Study the drawing (mm; zero at the part's minimum x, y, z) and answer. Round coordinates to 2 decimals unless told otherwise and drop trailing zeros. Loops run counter-clockwise (first coordinate to the right, second up) from the corner with the lowest first, then second, coordinate; pieces in that order, holes last. Notation, with made-up numbers: (58.25, -2) -> (71.25, -2) arc R26 cw to (71.25, 21) -> close; hole circle Ø4 at (-4, 17). An arc over 180 degrees is marked (long way). Write each question's results on one line, items separated by ' | '. Start each with the question number.
(1) The part is cut by section A-A (y = 2.5). Count the separate pieces of the cut face and the enclosed holes in it, plus the area to 3 significant figures.
(2) The part is cut by section D-D (z = 36). Determine the outline of the cut face in (x, y).
(3) The part is cut by section C-C (z = 12.7). Determine the outline of the cut face in (x, y).
(4) Straight lines are drawn through the part: probe 1 along X at (y, z) = (2, 38.1); probe 2 along Z at (x, y) = (19.5, 4.25) (1 decimal); probe 3 along Z at (x, y) = (21.5, 5.5) (1 decimal). For each, find the intervals that lie inside material, in ascending order.
(5) Determine the mould class of the marked faces 1 and 2 for opening direction X: released by +X, released by -X, zero draft, split by the parting line, or undercut.
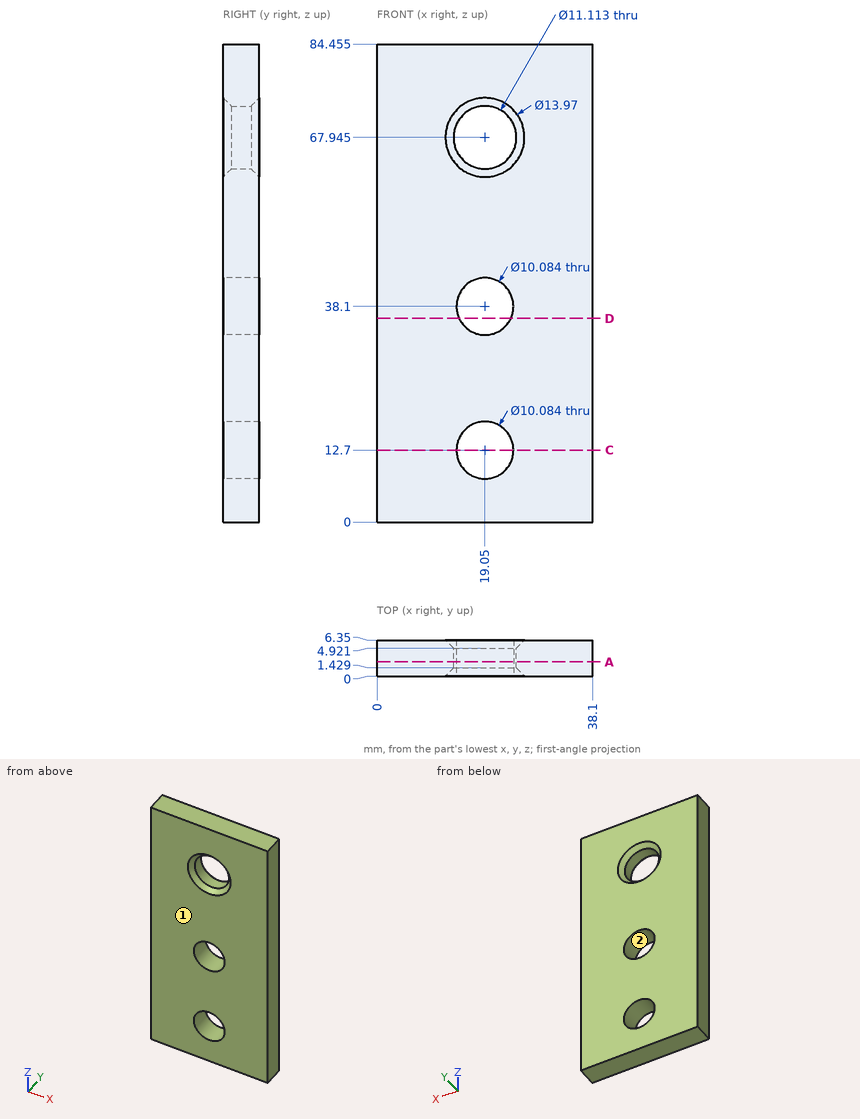
Checked values:
1) separate pieces: 1 | enclosed holes: 3 | area: 2,960 mm2
2) outline: (0, 0) -> (14.47, 0) -> (14.47, 6.35) -> (0, 6.35) -> close; (23.63, 0) -> (38.1, 0) -> (38.1, 6.35) -> (23.63, 6.35) -> close
3) outline: (0, 0) -> (14.01, 0) -> (14.01, 6.35) -> (0, 6.35) -> close; (24.09, 0) -> (38.1, 0) -> (38.1, 6.35) -> (24.09, 6.35) -> close
4) probe 1: x = 0 to 14.01, 24.09 to 38.1 | probe 2: z = 0 to 7.7, 17.7 to 33.1, 43.1 to 62.4, 73.5 to 84.5 | probe 3: z = 0 to 8.3, 17.1 to 33.7, 42.5 to 62.3, 73.6 to 84.5
5) face 1: zero draft | face 2: undercut
